from build123d import *

# Parameters (mm, degrees)
SCHIZZO1_W                   = 68
SCHIZZO1_H                   = 48
SCHIZZO1_R                   = 1.5
SCHIZZO1_R_2                 = 2.25
ESTRUSIONE_ESTRUSIONE1_DEPTH = 3
SCHIZZO2_W                   = 68
SCHIZZO2_H                   = 48
SCHIZZO2_R                   = 1.5
ESTRUSIONE_ESTRUSIONE2_DEPTH = 20
SCHIZZO3_W                   = 68
SCHIZZO3_H                   = 48
SCHIZZO3_W_2                 = 62
SCHIZZO3_H_2                 = 42
ESTRUSIONE_ESTRUSIONE3_DEPTH = 3
SMUSSO1_SIZE                 = 0.5
RACCORDO1_R                  = 5
SCHIZZO4_R                   = 4.5
TAGLIO_ESTRUSIONE1_DEPTH     = 1.5
RACCORDO2_R                  = 5
RACCORDO3_R                  = 1
TAGLIO_ESTRUSIONE2_REACH     = 78.655
SCHIZZO5_W                   = 7
SCHIZZO5_H                   = 7
RACCORDO4_R                  = 2.5
RACCORDO5_R                  = 0.5


with BuildPart() as part:
    # Schizzo1 → Estrusione-Estrusione1 (new body)
    with BuildSketch(Plane.XY):
        Rectangle(SCHIZZO1_W, SCHIZZO1_H)
        with Locations((-28, 18.1)):
            Circle(SCHIZZO1_R, mode=Mode.SUBTRACT)
        with Locations((-28, -18.1)):
            Circle(SCHIZZO1_R, mode=Mode.SUBTRACT)
        with Locations((28, -18.1)):
            Circle(SCHIZZO1_R, mode=Mode.SUBTRACT)
        with Locations((28, 18.1)):
            Circle(SCHIZZO1_R, mode=Mode.SUBTRACT)
        with Locations((20, -10)):
            Circle(SCHIZZO1_R_2, mode=Mode.SUBTRACT)
        with Locations((20, 10)):
            Circle(SCHIZZO1_R_2, mode=Mode.SUBTRACT)
        with Locations((-20, 10)):
            Circle(SCHIZZO1_R_2, mode=Mode.SUBTRACT)
        with Locations((-20, -10)):
            Circle(SCHIZZO1_R_2, mode=Mode.SUBTRACT)
    extrude(amount=ESTRUSIONE_ESTRUSIONE1_DEPTH)

    # Schizzo2 → Estrusione-Estrusione2 (add)
    with BuildSketch(Plane.XY.offset(3)):
        Rectangle(SCHIZZO2_W, SCHIZZO2_H)
        with BuildLine():
            ThreePointArc((-31, 15.454248689), (-25.224419663, 15.219695538), (-25.245004537, 21))
            Line((-25.245004537, 21), (25.245004537, 21))
            ThreePointArc((25.245004537, 21), (25.224419663, 15.219695538), (31, 15.454248689))
            Line((31, 15.454248689), (31, -15.454248689))
            ThreePointArc((31, -15.454248689), (25.224419663, -15.219695538), (25.245004537, -21))
            Line((25.245004537, -21), (-25.245004537, -21))
            ThreePointArc((-25.245004537, -21), (-25.224419663, -15.219695538), (-31, -15.454248689))
            Line((-31, -15.454248689), (-31, 15.454248689))
        make_face(mode=Mode.SUBTRACT)
        with BuildLine():
            ThreePointArc((-30.754995463, 21), (-30.880304462, 20.875580337), (-31, 20.745751311))
            Line((-31, 20.745751311), (-31, 21))
            Line((-31, 21), (-30.754995463, 21))
        make_face(mode=Mode.SUBTRACT)
        with Locations((-28, 18.1)):
            Circle(SCHIZZO2_R, mode=Mode.SUBTRACT)
        with BuildLine():
            Line((-31, -21), (-31, -20.745751311))
            ThreePointArc((-31, -20.745751311), (-30.880304462, -20.875580337), (-30.754995463, -21))
            Line((-30.754995463, -21), (-31, -21))
        make_face(mode=Mode.SUBTRACT)
        with BuildLine():
            Line((31, -21), (30.754995463, -21))
            ThreePointArc((30.754995463, -21), (30.880304462, -20.875580337), (31, -20.745751311))
            Line((31, -20.745751311), (31, -21))
        make_face(mode=Mode.SUBTRACT)
        with BuildLine():
            Line((31, 21), (31, 20.745751311))
            ThreePointArc((31, 20.745751311), (30.880304462, 20.875580337), (30.754995463, 21))
            Line((30.754995463, 21), (31, 21))
        make_face(mode=Mode.SUBTRACT)
        with Locations((-28, -18.1)):
            Circle(SCHIZZO2_R, mode=Mode.SUBTRACT)
        with Locations((28, -18.1)):
            Circle(SCHIZZO2_R, mode=Mode.SUBTRACT)
        with Locations((28, 18.1)):
            Circle(SCHIZZO2_R, mode=Mode.SUBTRACT)
    extrude(amount=ESTRUSIONE_ESTRUSIONE2_DEPTH)

    # Schizzo3 → Estrusione-Estrusione3 (add)
    with BuildSketch(Plane.XY.offset(23)):
        Rectangle(SCHIZZO3_W, SCHIZZO3_H)
        Rectangle(SCHIZZO3_W_2, SCHIZZO3_H_2, mode=Mode.SUBTRACT)
    extrude(amount=ESTRUSIONE_ESTRUSIONE3_DEPTH)

    # Smusso1
    smusso1_edges = [part.edges().sort_by_distance(p)[0] for p in [
        (-29.5, 18.1, 23),
        (26.5, -18.1, 23),
        (-29.5, -18.1, 23),
        (26.5, 18.1, 23),
    ]]
    chamfer(smusso1_edges, length=SMUSSO1_SIZE)

    # Raccordo1
    raccordo1_edges = [part.edges().sort_by_distance(p)[0] for p in [
        (34, 24, 13),
        (34, -24, 13),
        (-34, -24, 13),
        (-34, 24, 13),
    ]]
    fillet(raccordo1_edges, radius=RACCORDO1_R)

    # Schizzo4 → Taglio-Estrusione1 (cut)
    with BuildSketch(Plane.XY.offset(3)):
        with Locations((-20, 10)):
            Circle(SCHIZZO4_R)
        with Locations((-20, -10)):
            Circle(SCHIZZO4_R)
        with Locations((20, -10)):
            Circle(SCHIZZO4_R)
        with Locations((20, 10)):
            Circle(SCHIZZO4_R)
    extrude(amount=-TAGLIO_ESTRUSIONE1_DEPTH, mode=Mode.SUBTRACT)

    # Raccordo2
    raccordo2_edges = [part.edges().sort_by_distance(p)[0] for p in [
        (-31, 15.454248689, 13),
        (-25.245004537, 21, 13),
        (25.245004537, 21, 13),
        (31, 15.454248689, 13),
        (31, -15.454248689, 13),
        (25.245004537, -21, 13),
        (-25.245004537, -21, 13),
        (-31, -15.454248689, 13),
    ]]
    fillet(raccordo2_edges, radius=RACCORDO2_R)

    # Raccordo3
    raccordo3_edges = [part.edges().sort_by_distance(p)[0] for p in [
        (31, -21, 14.5),
        (-31, -21, 14.5),
        (-31, 21, 14.5),
        (31, 21, 14.5),
    ]]
    fillet(raccordo3_edges, radius=RACCORDO3_R)

    # Schizzo5 → Taglio-Estrusione2 (cut, up to next)
    with BuildSketch(Plane.ZY.offset(34), mode=Mode.PRIVATE) as taglio_estrusione2_sk1:
        with Locations((22.5, 0)):
            Rectangle(SCHIZZO5_W, SCHIZZO5_H)
    taglio_estrusione2_tool1 = extrude(taglio_estrusione2_sk1.sketch, amount=-TAGLIO_ESTRUSIONE2_REACH, mode=Mode.PRIVATE) & part.part
    add(taglio_estrusione2_tool1.solids().sort_by_distance((-34, 0, 22.5))[0], mode=Mode.SUBTRACT)

    # Raccordo4
    raccordo4_edges = [part.edges().sort_by_distance(p)[0] for p in [
        (-31, -3.5, 22.5),
        (-31, 0, 19),
        (-31, 3.5, 22.5),
    ]]
    fillet(raccordo4_edges, radius=RACCORDO4_R)

    # Raccordo5
    raccordo5_edges = [part.edges().sort_by_distance(p)[0] for p in [
        (-34, -3.5, 22.5),
        (-34, 0, 19),
        (-34, 3.5, 22.5),
    ]]
    fillet(raccordo5_edges, radius=RACCORDO5_R - 0.0001)  # a hair under: the kernel refuses the full size


solid = part.part
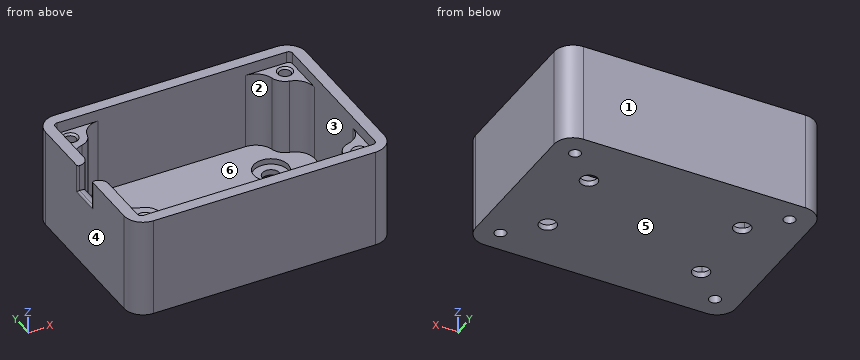
Can you work these out from the model? Positions are in its coordinate system, mm. Face numbers are marked on the shaded views. A direction names the side the tool comes from. Give positions to 0.01 mm unless a question says otherwise; leave off trailing zeros. Loops run counter-clockwise (first coordinate to the right, second up) from the corner with the lowest first, then second, coordinate; pieces in that order, holes last. Notation, with made-up numbers: (10, 60) -> (23, 60) arc R29 ccw to (23, 93) -> close; hole circle Ø4 at (55, -11). An arc over 180 degrees is marked (long way). Use one line per item in the form item = value.
1) Will these pins go through, and if not, where does the flat tip stop? pin 1 (7 mm diameter, centred on x = -19, y = 9.5, fed in from +Z); pin 2 (9.5 mm diameter, centred on x = 22.5, y = -16, fed in from +Z).
Answers:
pin_1 = 3
pin_2 = 23
2) If we section it at D-D (x = -28): Please give me the cut outline in (y, z).
Answers:
outline = (-24, 0) -> (-19.6, 0) -> (-19.6, 22.5) -> (-20.1, 23) -> (-21, 23) -> (-21, 26) -> (-24, 26) -> close; (-16.6, 0) -> (16.6, 0) -> (16.6, 22.5) -> (16.1, 23) -> (13.91, 23) -> (13.91, 3) -> (-13.91, 3) -> (-13.91, 23) -> (-16.1, 23) -> (-16.6, 22.5) -> close; (19.6, 0) -> (24, 0) -> (24, 26) -> (21, 26) -> (21, 23) -> (20.1, 23) -> (19.6, 22.5) -> close
3) If we section it at A-A (z = 14.5): Please give me the cut outline in (x, y), plus the area to 3 significant figures.
Answers:
outline = (-34, -19) arc R5 ccw to (-29, -24) -> (29, -24) arc R5 ccw to (34, -19) -> (34, 19) arc R5 ccw to (29, 24) -> (-29, 24) arc R5 ccw to (-34, 19) -> close; hole (-31, -9.33) arc R5 ccw to (-27.11, -14.2) arc R4 cw to (-24.11, -17.17) arc R5 ccw to (-19.25, -21) -> (19.25, -21) arc R5 ccw to (24.11, -17.17) arc R4 cw to (27.11, -14.2) arc R5 ccw to (31, -9.33) -> (31, 9.33) arc R5 ccw to (27.11, 14.2) arc R4 cw to (24.11, 17.17) arc R5 ccw to (19.25, 21) -> (-19.25, 21) arc R5 ccw to (-24.11, 17.17) arc R4 cw to (-27.11, 14.2) arc R5 ccw to (-31, 9.33) -> close; hole circle Ø3 at (-28, -18.1); hole circle Ø3 at (-28, 18.1); hole circle Ø3 at (28, -18.1); hole circle Ø3 at (28, 18.1)
area = 825 mm²
4) If we section it at B-B (x = -1): Please give me the cut outline in (y, z).
Answers:
outline = (-24, 0) -> (24, 0) -> (24, 26) -> (21, 26) -> (21, 3) -> (-21, 3) -> (-21, 26) -> (-24, 26) -> close
5) We'd pull the mould along X, two halves only. Please class the marked faces 3, 4, 5 and 6: released by +X, released by -X, zero draft, split by the parting line, or undercut.
Answers:
face_3 = undercut
face_4 = released by -X
face_5 = zero draft
face_6 = undercut
6) For the marked faces 1 and 2, which set-ups out of +Z, -Z, +X, -X, +Y, -Y let a thin tool reach every point of the face, with its end or its side?
Answers:
face_1 = +Z, -Z, +X, -X, +Y
face_2 = +Z
7) If we section it at C-C (y = 18.1): Please give me the cut outline in (x, z), plus the area to 3 significant figures.
Answers:
outline = (-34, 0) -> (-29.5, 0) -> (-29.5, 22.5) -> (-30, 23) -> (-31, 23) -> (-31, 26) -> (-34, 26) -> close; (-26.5, 0) -> (26.5, 0) -> (26.5, 22.5) -> (26, 23) -> (23.79, 23) -> (23.79, 3) -> (-23.79, 3) -> (-23.79, 23) -> (-26, 23) -> (-26.5, 22.5) -> close; (29.5, 0) -> (34, 0) -> (34, 26) -> (31, 26) -> (31, 23) -> (30, 23) -> (29.5, 22.5) -> close
area = 492 mm²
8) I need wall thicknesses on line 1 along X through (y, z) = (10, 1.1); line 2 along X through (y, z) = (2, 15.5); line 3 along Y through (x, z) = (28, 11.5). Which ranges of each line are inside material? Lowest first, please.
Answers:
line_1 = -34 to -22.25, -17.75 to 17.75, 22.25 to 34
line_2 = -34 to -31, 31 to 34
line_3 = -24 to -19.6, -16.6 to -13.91, 13.91 to 16.6, 19.6 to 24
